Autodesk Inventor part; units mm, degrees
ref_plane "YZ Plane" through (0, 0, 0) normal (1, 0, 0) x (0, 1, 0)
ref_plane "XZ Plane" through (0, 0, 0) normal (0, 1, 0) x (-1, 0, 0)
ref_plane "XY Plane" through (0, 0, 0) normal (0, 0, 1) x (1, 0, 0)
sketch "Sketch1" plane through (0, 0, 0) normal (0, 1, 0) x (-1, 0, 0)
  line L0 (19.7891, 28.4759) -> (-41.5109, 28.4759)
  line L1 (-41.5109, 28.4759) -> (-41.5109, -21.3241)
  line L2 (-41.5109, -21.3241) -> (19.7891, -21.3241)
  line L3 (19.7891, -21.3241) -> (19.7891, 28.4759)
  point P0 (0, 0)
  dimension "d0" = 49.8
  dimension "d1" = 61.3
extrude "Extrusion1" add sketch "Sketch1" along normal blind 9.3
sketch "Sketch2" plane through (0, 9.3, 0) normal (0, 1, 0) x (1, 0, 0)
  line L0 (-18.7891, 20.3241) -> (40.5109, 20.3241)
  line L1 (40.5109, 20.3241) -> (40.5109, -27.4759)
  line L2 (40.5109, -27.4759) -> (-18.7891, -27.4759)
  line L3 (-18.7891, -27.4759) -> (-18.7891, 20.3241)
  line L4 (41.5109, 21.3241) -> (-19.7891, 21.3241)
  line L5 (-19.7891, 21.3241) -> (-19.7891, -28.4759)
  point P0 (0, 0)
  dimension "d4" = 59.3
  dimension "d5" = 47.8
  dimension "d6" = 1
  dimension "d7" = 1
extrude "Extrusion2" cut sketch "Sketch2" against normal blind 8
sketch "Sketch3" plane through (0, 1.3, 0) normal (0, 1, 0) x (1, 0, 0)
  line L0 (-18.7891, 20.3241) -> (40.5109, 20.3241)
  line L1 (40.5109, -27.4759) -> (-18.7891, -27.4759)
  line L2 (-18.7891, 20.3241) -> (-17.7891, 20.3241)
  line L3 (-17.7891, 20.3241) -> (-17.7891, -27.4759)
  line L4 (-17.7891, -27.4759) -> (-18.7891, -27.4759)
  line L5 (-18.7891, -27.4759) -> (-18.7891, 20.3241)
  line L6 (-4.7891, 20.3241) -> (-5.7891, 20.3241)
  line L7 (-5.7891, 20.3241) -> (-5.7891, -27.4759)
  line L8 (-5.7891, -27.4759) -> (-4.7891, -27.4759)
  line L9 (-4.7891, -27.4759) -> (-4.7891, 20.3241)
  line L10 (-17.7891, 8.3241) -> (-5.7891, 8.3241)
  line L11 (-5.7891, 8.3241) -> (-5.7891, 7.3241)
  line L12 (-5.7891, 7.3241) -> (-17.7891, 7.3241)
  line L13 (-17.7891, 7.3241) -> (-17.7891, 8.3241)
  line L14 (-17.7891, -2.9259) -> (-5.7891, -2.9259)
  line L15 (-5.7891, -2.9259) -> (-5.7891, -3.9259)
  line L16 (-5.7891, -3.9259) -> (-17.7891, -3.9259)
  line L17 (-17.7891, -3.9259) -> (-17.7891, -2.9259)
  line L18 (-17.7891, -14.1759) -> (-5.7891, -14.1759)
  line L19 (-5.7891, -14.1759) -> (-5.7891, -15.1759)
  line L20 (-5.7891, -15.1759) -> (-17.7891, -15.1759)
  line L21 (-17.7891, -15.1759) -> (-17.7891, -14.1759)
  line L22 (-19.7891, 21.3241) -> (-19.7891, -28.4759)
  line L23 (-17.7891, 20.3241) -> (-5.7891, 20.3241)
  line L24 (-5.7891, 20.3241) -> (-5.7891, 19.3241)
  line L25 (-5.7891, 19.3241) -> (-17.7891, 19.3241)
  line L26 (-17.7891, 19.3241) -> (-17.7891, 20.3241)
  line L27 (-17.7891, -26.4759) -> (-5.7891, -26.4759)
  line L28 (-5.7891, -26.4759) -> (-5.7891, -27.4759)
  line L29 (-5.7891, -27.4759) -> (-17.7891, -27.4759)
  line L30 (-17.7891, -27.4759) -> (-17.7891, -26.4759)
  line L31 (5.5109, 19.3241) -> (-6.4891, 19.3241)
  line L32 (6.5109, -27.4759) -> (6.5109, 20.3241)
  line L33 (5.5109, 20.3241) -> (5.5109, -27.4759)
  line L34 (-6.4891, 8.3241) -> (5.5109, 8.3241)
  line L35 (5.5109, 7.3241) -> (-6.4891, 7.3241)
  line L36 (-6.4891, -2.9259) -> (5.5109, -2.9259)
  line L37 (5.5109, -3.9259) -> (-6.4891, -3.9259)
  line L38 (-6.4891, -14.1759) -> (5.5109, -14.1759)
  line L39 (5.5109, -15.1759) -> (-6.4891, -15.1759)
  line L40 (-6.4891, -26.4759) -> (5.5109, -26.4759)
  line L41 (5.5109, -27.4759) -> (-6.4891, -27.4759)
  line L42 (16.8109, 19.3241) -> (4.8109, 19.3241)
  line L43 (17.8109, -27.4759) -> (17.8109, 20.3241)
  line L44 (16.8109, 20.3241) -> (16.8109, -27.4759)
  line L45 (4.8109, 8.3241) -> (16.8109, 8.3241)
  line L46 (16.8109, 7.3241) -> (4.8109, 7.3241)
  line L47 (4.8109, -2.9259) -> (16.8109, -2.9259)
  line L48 (16.8109, -3.9259) -> (4.8109, -3.9259)
  line L49 (4.8109, -14.1759) -> (16.8109, -14.1759)
  line L50 (16.8109, -15.1759) -> (4.8109, -15.1759)
  line L51 (4.8109, -26.4759) -> (16.8109, -26.4759)
  line L52 (16.8109, -27.4759) -> (4.8109, -27.4759)
  line L53 (28.1109, 19.3241) -> (16.1109, 19.3241)
  line L54 (29.1109, -27.4759) -> (29.1109, 20.3241)
  line L55 (28.1109, 20.3241) -> (28.1109, -27.4759)
  line L56 (16.1109, 8.3241) -> (28.1109, 8.3241)
  line L57 (28.1109, 7.3241) -> (16.1109, 7.3241)
  line L58 (16.1109, -2.9259) -> (28.1109, -2.9259)
  line L59 (28.1109, -3.9259) -> (16.1109, -3.9259)
  line L60 (16.1109, -14.1759) -> (28.1109, -14.1759)
  line L61 (28.1109, -15.1759) -> (16.1109, -15.1759)
  line L62 (16.1109, -26.4759) -> (28.1109, -26.4759)
  line L63 (28.1109, -27.4759) -> (16.1109, -27.4759)
  line L64 (39.4109, 19.3241) -> (27.4109, 19.3241)
  line L65 (40.4109, -27.4759) -> (40.4109, 20.3241)
  line L66 (39.4109, 20.3241) -> (39.4109, -27.4759)
  line L67 (27.4109, 8.3241) -> (39.4109, 8.3241)
  line L68 (39.4109, 7.3241) -> (27.4109, 7.3241)
  line L69 (27.4109, -2.9259) -> (39.4109, -2.9259)
  line L70 (39.4109, -3.9259) -> (27.4109, -3.9259)
  line L71 (27.4109, -14.1759) -> (39.4109, -14.1759)
  line L72 (39.4109, -15.1759) -> (27.4109, -15.1759)
  line L73 (27.4109, -26.4759) -> (39.4109, -26.4759)
  line L74 (39.4109, -27.4759) -> (27.4109, -27.4759)
  point P0 (0, 0)
  point P1 (-11.7891, 8.3241)
  point P2 (-0.4891, 8.3241)
  point P3 (10.8109, 8.3241)
  point P4 (22.1109, 8.3241)
  point P5 (33.4109, 8.3241)
  point P6 (-18.7891, -27.4759)
  point P7 (40.4109, 20.3241)
  point P8 (17.8109, 20.3241)
  point P9 (17.8109, 19.3241)
  point P10 (17.8109, 8.3241)
  point P11 (6.5109, 8.3241)
  point P12 (6.5109, 19.3241)
  point P13 (-4.7891, 19.3241)
  point P14 (-4.7891, 8.3241)
  point P15 (-4.7891, 7.3241)
  point P16 (-4.7891, -2.9259)
  point P17 (-4.7891, -3.9259)
  point P18 (-4.7891, -14.1759)
  point P19 (6.5109, -3.9259)
  point P20 (6.5109, -14.1759)
  point P21 (17.8109, 7.3241)
  point P22 (17.8109, -2.9259)
  point P23 (17.8109, -15.1759)
  point P24 (17.8109, -26.4759)
  point P25 (29.1109, -2.9259)
  point P26 (29.1109, 7.3241)
  point P27 (29.1109, -26.4759)
  point P28 (29.1109, -15.1759)
  point P29 (29.1109, -14.1759)
  point P30 (29.1109, -3.9259)
  point P31 (29.1109, 19.3241)
  point P32 (29.1109, 8.3241)
  point P33 (17.8109, -3.9259)
  point P34 (17.8109, -14.1759)
  point P35 (6.5109, -15.1759)
  point P36 (6.5109, -26.4759)
  point P37 (6.5109, 7.3241)
  point P38 (6.5109, -2.9259)
  point P39 (-4.7891, -15.1759)
  point P40 (-4.7891, -26.4759)
  dimension "d10" = 1
  dimension "d12" = 1
  dimension "d13" = 12
  dimension "d14" = 1
  dimension "d15" = 12
  dimension "d16" = 1
  dimension "d17" = 1
  dimension "d18" = 10.25
  dimension "d19" = 10.25
  dimension "d20" = 2
  dimension "d21" = 1
  dimension "d22" = 1
  dimension "d25" = 11.3
extrude "Extrusion3" add sketch "Sketch3" along normal blind 0.2 contours L0 L3 L1 L5 | L0 L7 L25 L3 | L0 L9 L31 L7 | L3 L27 L7 L1 | L0 L33 L31 L9 | L31 L9 L34 L7 | L10 L7 L12 L3 | L0 L32 L42 L33 | L34 L9 L35 L7 | L7 L40 L9 L1 | L3 L18 L7 L20 | L0 L44 L42 L32 | L42 L32 L45 L33 | L34 L33 L35 L9 | L35 L9 L36 L7 | L14 L7 L16 L3 | L9 L40 L33 L1 | L7 L39 L9 L40 | L45 L32 L46 L33 | L36 L9 L37 L7 | L7 L38 L9 L39 | L0 L55 L53 L43 | L53 L43 L56 L44 | L45 L44 L46 L32 | L46 L32 L47 L33 | L36 L33 L37 L9 | L37 L9 L38 L7 | L33 L51 L32 L1 | L9 L38 L33 L39 | L0 L54 L64 L55 | L56 L43 L57 L44 | L47 L32 L48 L33 | L32 L51 L44 L1 | L33 L50 L32 L51 | L0 L66 L64 L54 | L64 L54 L67 L55 | L56 L55 L57 L43 | L57 L43 L58 L44 | L47 L44 L48 L32 | L48 L32 L49 L33 | L33 L49 L32 L50 | L0 L65 L1 L66 | L67 L54 L68 L55 | L58 L43 L59 L44 | L44 L62 L43 L1 | L32 L49 L44 L50 | L67 L66 L68 L54 | L68 L54 L69 L55 | L58 L55 L59 L43 | L59 L43 L60 L44 | L43 L62 L55 L1 | L44 L61 L43 L62 | L69 L54 L70 L55 | L60 L43 L61 L44 | L1 L54 L73 L66 | L69 L66 L70 L54 | L70 L54 L71 L55 | L60 L55 L61 L43 | L55 L73 L54 L1 | L71 L54 L72 L55 | L55 L72 L54 L73 | L72 L54 L71 L66
properties part number "PanHolderLid"
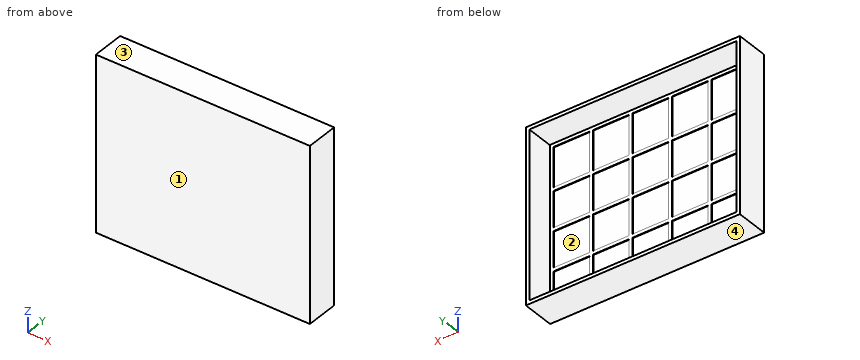
Verification items for the finished model (mm, model axes). Face numbers are marked on the shaded views. Give positions to 0.01 mm unless a question says otherwise; leave off trailing zeros. Write each loop counter-clockwise with the first axis right and the second up, starting at its lowest first coordinate (ties: lowest second). Pieces come first, ordered by that corner, then holes. Notation, with made-up numbers: M 31,-11.5 L 54,-11.5 A6 ccw 54,-4.5 Z; hole C -13,-8 d9. An arc over 180 degrees is marked long. Use CSV: the item, a comma, the result in double quotes.
1) Release check for a two-part mould opening along Z. For the marked faces 1, 2, 3 and 4 record: released by +Z, released by -Z, zero draft, split by the parting line, or undercut.
Final values:
face 1,"zero draft"
face 2,"undercut"
face 3,"released by +Z"
face 4,"released by -Z"
2) Cross-section at B-B (x = 4). Enter the section's corners in (y, z).
Final values:
outline,"M 0,-21.32 L 9.3,-21.32 L 9.3,-20.32 L 1.5,-20.32 L 1.5,-19.32 L 1.3,-19.32 L 1.3,-8.32 L 1.5,-8.32 L 1.5,-7.32 L 1.3,-7.32 L 1.3,2.93 L 1.5,2.93 L 1.5,3.93 L 1.3,3.93 L 1.3,14.18 L 1.5,14.18 L 1.5,15.18 L 1.3,15.18 L 1.3,26.48 L 1.5,26.48 L 1.5,27.48 L 9.3,27.48 L 9.3,28.48 L 0,28.48 Z"
3) Material ranges on line 1 along X through (y, z) = (7.75, 8); line 2 along Z through (x, y) = (22, 5.25); line 3 along Y through (x, z) = (28.5, 22), recorded low to high.
Final values:
line 1,"-19.79 to -18.79, 40.51 to 41.51"
line 2,"-21.32 to -20.32, 27.48 to 28.48"
line 3,"0 to 1.5"
4) Go/stop test with flat-tipped pins: pin 1 Ø1 at (x, z) = (26.5, 0.5) entering from +Y; pin 2 Ø8 at (x, z) = (-1.5, -15.5) entering from +Y. Record where each tip stops, or that it passes through.
Final values:
pin 1,"y = 1.3"
pin 2,"y = 1.5"
5) Cross-section at A-A (y = 3.25). Enter the section's corners in (x, z), plus the area to 3 significant figures.
Final values:
outline,"M -19.79,-21.32 L 41.51,-21.32 L 41.51,28.48 L -19.79,28.48 Z; hole M -18.79,-20.32 L 40.51,-20.32 L 40.51,27.48 L -18.79,27.48 Z"
area,"218 mm²"
